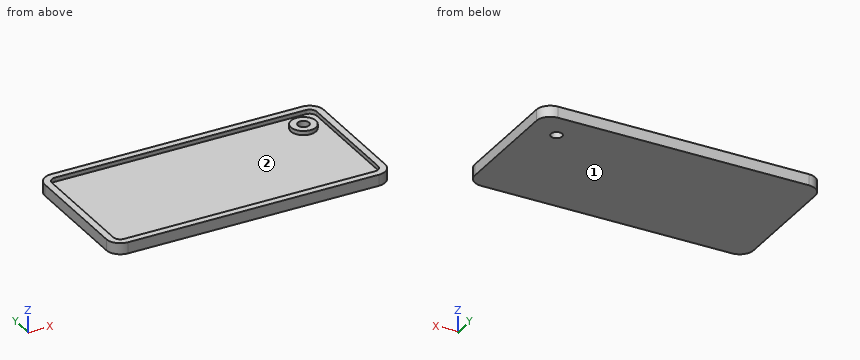
from build123d import *

# Parameters (mm, degrees)
F1_DEPTH = 4
F2_D     = 4
F3_T     = -2.5


with BuildPart() as f1:
    # F0 (on Top) → F1 (new body)
    with BuildSketch(Plane.XY):
        with BuildLine():
            ThreePointArc((0, 5), (1.4644660941, 1.4644660941), (5, 0))
            Line((5, 0), (95, 0))
            ThreePointArc((95, 0), (98.5355339059, 1.4644660941), (100, 5))
            Line((100, 5), (100, 45))
            ThreePointArc((100, 45), (98.5355339059, 48.5355339059), (95, 50))
            Line((95, 50), (5, 50))
            ThreePointArc((5, 50), (1.4644660941, 48.5355339059), (0, 45))
            Line((0, 45), (0, 5))
        make_face()
        with BuildLine():
            ThreePointArc((5, 40), (6.4644660941, 43.5355339059), (10, 45))
            Line((10, 45), (90, 45))
            ThreePointArc((90, 45), (93.5355339059, 43.5355339059), (95, 40))
            Line((95, 40), (95, 10))
            ThreePointArc((95, 10), (93.5355339059, 6.4644660941), (90, 5))
            Line((90, 5), (10, 5))
            ThreePointArc((10, 5), (6.4644660941, 6.4644660941), (5, 10))
            Line((5, 10), (5, 40))
        make_face(mode=Mode.SUBTRACT)
        with BuildLine():
            Line((90, 45), (10, 45))
            ThreePointArc((10, 45), (6.4644660941, 43.5355339059), (5, 40))
            Line((5, 40), (5, 10))
            ThreePointArc((5, 10), (6.4644660941, 6.4644660941), (10, 5))
            Line((10, 5), (90, 5))
            ThreePointArc((90, 5), (93.5355339059, 6.4644660941), (95, 10))
            Line((95, 10), (95, 40))
            ThreePointArc((95, 40), (93.5355339059, 43.5355339059), (90, 45))
        make_face()
    extrude(amount=F1_DEPTH)

    # F2 (through all)
    with Locations(Plane(origin=(0, 0, 0), x_dir=(1, 0, 0), z_dir=(0, 0, -1))):
        with Locations((90, -40)):
            Hole(F2_D / 2)

    # F3
    f3_openings = [f1.faces().sort_by_distance(p)[0] for p in [
        (49.89878, 24.962043, 4),
    ]]
    offset(amount=F3_T, openings=f3_openings)


solid = f1.part
Model file for the job. Use its own axes, mm. Face numbers are marked on the shaded views. Round coordinates to 2 decimals unless told otherwise and drop trailing zeros. Loops run counter-clockwise (first coordinate to the right, second up) from the corner with the lowest first, then second, coordinate; pieces in that order, holes last. Notation, with made-up numbers: (-27, 25.25) -> (28, 25.25) arc R21 cw to (28, 39.25) -> close; hole circle Ø3 at (-17.5, -5). An arc over 180 degrees is marked (long way). Answer as CSV lines item,"result". Start each with the question number.
1) Slice it at C-C (y = 40). List the corners of the cut face in (x, z).
2) Slice it at A-A (x = 90). List the corners of the cut face in (y, z), plus the area to 3 significant figures.
3) Pin check, flat tips, straight feed: P1, Ø1.5, axis at y = 18, z = 2, coming from the -X side; P2, Ø4, axis at x = 50.5, y = 43.5, coming from the +Z side. Stop position of each tip, or through.
4) Mould opens along X. For the marked faces 1 and 2 say: +X half, -X half, draft (parallel to the pull), parting line (faces both ways), or undercut.
5) Probe line 1 along X through (y, z) = (40, 1); line 2 along X through (y, z) = (40, 2.7); line 3 along X through (y, z) = (29.5, 3.6). List the from-to ranges inside material, lowest first.
6) Slice it at B-B (z = 3.2). List the corners of the cut face in (x, y).
7) Slice it at D-D (x = 53). List the corners of the cut face in (y, z).
Filled in:
1,outline,"(0, 0) -> (88, 0) -> (88, 4) -> (85.5, 4) -> (85.5, 2.5) -> (2.5, 2.5) -> (2.5, 4) -> (0, 4) -> close; (92, 0) -> (100, 0) -> (100, 4) -> (97.5, 4) -> (97.5, 2.5) -> (94.5, 2.5) -> (94.5, 4) -> (92, 4) -> close"
2,outline,"(0, 0) -> (38, 0) -> (38, 4) -> (35.5, 4) -> (35.5, 2.5) -> (2.5, 2.5) -> (2.5, 4) -> (0, 4) -> close; (42, 0) -> (50, 0) -> (50, 4) -> (47.5, 4) -> (47.5, 2.5) -> (44.5, 2.5) -> (44.5, 4) -> (42, 4) -> close"
2,area,"130 mm2"
3,P1,"stops at x = 0"
3,P2,"stops at z = 2.5"
4,face 1,"draft"
4,face 2,"undercut"
5,line 1,"x = 0 to 88, 92 to 100"
5,line 2,"x = 0 to 2.5, 85.5 to 88, 92 to 94.5, 97.5 to 100"
5,line 3,"x = 0 to 2.5, 97.5 to 100"
6,outline,"(0, 5) arc R5 ccw to (5, 0) -> (95, 0) arc R5 ccw to (100, 5) -> (100, 45) arc R5 ccw to (95, 50) -> (5, 50) arc R5 ccw to (0, 45) -> close; circle Ø9 at (90, 40); hole (2.5, 5) arc R2.5 ccw to (5, 2.5) -> (95, 2.5) arc R2.5 ccw to (97.5, 5) -> (97.5, 45) arc R2.5 ccw to (95, 47.5) -> (5, 47.5) arc R2.5 ccw to (2.5, 45) -> close; hole circle Ø4 at (90, 40)"
7,outline,"(0, 0) -> (50, 0) -> (50, 4) -> (47.5, 4) -> (47.5, 2.5) -> (2.5, 2.5) -> (2.5, 4) -> (0, 4) -> close"
